from build123d import *

# Parameters (mm, degrees)
BOSS_EXTRUDE1_DEPTH = 15
SKETCH2_R           = 3.5
CUT_EXTRUDE1_DEPTH  = 11
CUT_EXTRUDE2_REACH  = 59.639
SKETCH3_R           = 2
SKETCH4_R           = 2
BOSS_EXTRUDE5_DEPTH = 4


with BuildPart() as part:
    # Sketch1 → Boss-Extrude1 (new body)
    with BuildSketch(Plane.XY):
        Polygon((0, 0), (0, 20.5), (41, 20.5), (41, 0), (51, 0), (51, 24.5), (-10, 24.5), (-10, 0), align=None)
    extrude(amount=BOSS_EXTRUDE1_DEPTH)

    # Sketch2 → Cut-Extrude1 (cut)
    with BuildSketch(Plane.XY.offset(15)):
        with Locations((45, 5)):
            Circle(SKETCH2_R)
        with Locations((45, 15)):
            Circle(SKETCH2_R)
        with Locations((-4, 5)):
            Circle(SKETCH2_R)
        with Locations((-4, 15)):
            Circle(SKETCH2_R)
    extrude(amount=-CUT_EXTRUDE1_DEPTH, mode=Mode.SUBTRACT)

    # Sketch3 → Cut-Extrude2 (cut, up to next)
    with BuildSketch(Plane.XY.offset(4), mode=Mode.PRIVATE) as cut_extrude2_sk1:
        with Locations((-4, 15)):
            Circle(SKETCH3_R)
    cut_extrude2_tool1 = extrude(cut_extrude2_sk1.sketch, amount=-CUT_EXTRUDE2_REACH, mode=Mode.PRIVATE) & part.part
    # Sketch3 → Cut-Extrude2 (cut, up to next)
    with BuildSketch(Plane.XY.offset(4), mode=Mode.PRIVATE) as cut_extrude2_sk2:
        with Locations((-4, 5)):
            Circle(SKETCH3_R)
    cut_extrude2_tool2 = extrude(cut_extrude2_sk2.sketch, amount=-CUT_EXTRUDE2_REACH, mode=Mode.PRIVATE) & part.part
    # Sketch3 → Cut-Extrude2 (cut, up to next)
    with BuildSketch(Plane.XY.offset(4), mode=Mode.PRIVATE) as cut_extrude2_sk3:
        with Locations((45, 15)):
            Circle(SKETCH3_R)
    cut_extrude2_tool3 = extrude(cut_extrude2_sk3.sketch, amount=-CUT_EXTRUDE2_REACH, mode=Mode.PRIVATE) & part.part
    # Sketch3 → Cut-Extrude2 (cut, up to next)
    with BuildSketch(Plane.XY.offset(4), mode=Mode.PRIVATE) as cut_extrude2_sk4:
        with Locations((45, 5)):
            Circle(SKETCH3_R)
    cut_extrude2_tool4 = extrude(cut_extrude2_sk4.sketch, amount=-CUT_EXTRUDE2_REACH, mode=Mode.PRIVATE) & part.part
    add(cut_extrude2_tool1.solids().sort_by_distance((-4, 15, 4))[0], mode=Mode.SUBTRACT)
    add(cut_extrude2_tool2.solids().sort_by_distance((-4, 5, 4))[0], mode=Mode.SUBTRACT)
    add(cut_extrude2_tool3.solids().sort_by_distance((45, 15, 4))[0], mode=Mode.SUBTRACT)
    add(cut_extrude2_tool4.solids().sort_by_distance((45, 5, 4))[0], mode=Mode.SUBTRACT)

    # Sketch4 → Boss-Extrude5 (add)
    # profile 1 of 2: a face of its own
    with BuildSketch(Plane.XZ):
        with BuildLine():
            Line((51, 1.5), (58, 1.5))
            ThreePointArc((58, 1.5), (64, 7.5), (58, 13.5))
            Line((58, 13.5), (51, 13.5))
            Line((51, 13.5), (51, 1.5))
        make_face()
        with Locations(Location((58, 7.5, 0), (0, 0, 270))):
            Circle(SKETCH4_R, mode=Mode.SUBTRACT)
    # profile 2 of 2: a face of its own
    with BuildSketch(Plane.XZ):
        with BuildLine():
            ThreePointArc((-17, 13.5), (-23, 7.5), (-17, 1.5))
            Line((-17, 1.5), (-10, 1.5))
            Line((-10, 1.5), (-10, 13.5))
            Line((-10, 13.5), (-17, 13.5))
        make_face()
        with Locations(Location((-17, 7.5, 0), (0, 0, 270))):
            Circle(SKETCH4_R, mode=Mode.SUBTRACT)
    extrude(amount=-BOSS_EXTRUDE5_DEPTH)


solid = part.part
For this review, take the finished solid that the model builds, in its own axes (mm). A direction names the side the tool comes from. Give positions to 0.01 mm unless a question says otherwise; leave off trailing zeros. Loops run counter-clockwise (first coordinate to the right, second up) from the corner with the lowest first, then second, coordinate; pieces in that order, holes last.
Item 1: Insertion check: pin 1 (5.5 mm diameter, centred on x = 45, y = 15, fed in from +Z); pin 2 (4.5 mm diameter, centred on y = 18, z = 11, fed in from +X); pin 3 (3.5 mm diameter, centred on x = 58.5, z = 7, fed in from +Y). Each pin has a flat end and moves straight along its axis. Give the tip position at first contact, or say it passes through.
Item 2: Take a section at A-A, the plane x = -4. State the section outline as (y, z) points.
Item 3: Take a section at C-C, the plane z = 7.5. State the section outline as (x, y) points.
Item 4: Take a section at B-B, the plane y = 15. State the section outline as (x, z) points, and give its area (3 significant figures).
Item 5: Take a section at D-D, the plane z = 12. State the section outline as (x, y) points.
Item 6: For line 1 along Y through (x, z) = (45, 1.9); line 2 along Y through (x, z) = (45, 9.25); line 3 along X through (y, z) = (2.35, 7.5), list the stretches that pass through material, from the lowest coordinate up.
Item 7: Tool access review of faces 4 (the flat face through (55, 2, 13.5)), 5 (the flat face through (20, 20.5, 7)), 6 (the flat face through (54, 2, 1.5)), 7 (the cylindrical face through (41.503, 15.154, 9.577)): name each direction out of +Z, -Z, +X, -X, +Y, -Y from which nothing blocks a thin tool from reaching the whole face with its end or side.
Item 8: Draft analysis for pull direction Y (two halves, no side actions). For faces 1 (the flat face through (50, 0, 7)), 2 (the cylindrical face through (-4, 17, 2)), 3 (the flat face through (0, 10, 7)), state which applies: +Y half, -Y half, draft (parallel to the pull), parting line (faces both ways), or undercut.
Calculated:
1. pin 1: stops at z = 4
1. pin 2: stops at x = 51
1. pin 3: stops at y = 4
2. outline: (0, 0) - (3, 0) - (3, 4) - (1.5, 4) - (1.5, 15) - (0, 15) - close; (7, 0) - (13, 0) - (13, 4) - (11.5, 4) - (11.5, 15) - (8.5, 15) - (8.5, 4) - (7, 4) - close; (17, 0) - (24.5, 0) - (24.5, 15) - (18.5, 15) - (18.5, 4) - (17, 4) - close
3. outline: (-23, 0) - (-19, 0) - (-19, 4) - (-23, 4) - close; (-15, 0) - (0, 0) - (0, 20.5) - (41, 20.5) - (41, 0) - (56, 0) - (56, 4) - (51, 4) - (51, 24.5) - (-10, 24.5) - (-10, 4) - (-15, 4) - close; (60, 0) - (64, 0) - (64, 4) - (60, 4) - close; hole circle Ø7 at (-4, 5); hole circle Ø7 at (-4, 15); hole circle Ø7 at (45, 5); hole circle Ø7 at (45, 15)
4. outline: (-10, 0) - (-6, 0) - (-6, 4) - (-7.5, 4) - (-7.5, 15) - (-10, 15) - close; (-2, 0) - (0, 0) - (0, 15) - (-0.5, 15) - (-0.5, 4) - (-2, 4) - close; (41, 0) - (43, 0) - (43, 4) - (41.5, 4) - (41.5, 15) - (41, 15) - close; (47, 0) - (51, 0) - (51, 15) - (48.5, 15) - (48.5, 4) - (47, 4) - close
4. area: 114 mm2
5. outline: (-20.97, 0) - (0, 0) - (0, 20.5) - (41, 20.5) - (41, 0) - (61.97, 0) - (61.97, 4) - (51, 4) - (51, 24.5) - (-10, 24.5) - (-10, 4) - (-20.97, 4) - close; hole circle Ø7 at (-4, 5); hole circle Ø7 at (-4, 15); hole circle Ø7 at (45, 5); hole circle Ø7 at (45, 15)
6. line 1: y = 0 to 3, 7 to 13, 17 to 24.5
6. line 2: y = 0 to 1.5, 8.5 to 11.5, 18.5 to 24.5
6. line 3: x = -23 to -19, -15 to -6.29, -1.71 to 0, 41 to 42.71, 47.29 to 56, 60 to 64
7. face 4: +Z, +X, +Y, -Y
7. face 5: +Z, -Z, -Y
7. face 6: -Z, +X, +Y, -Y
7. face 7: +Z
8. face 1: -Y half
8. face 2: undercut
8. face 3: draft
